from build123d import *

# Parameters (mm, degrees)
F0_W     = 62
F0_H     = 78
F0_W_2   = 8
F0_H_2   = 5
F1_DEPTH = 20
F2_W     = 54.3611720204
F2_H     = 31.5054729581
F3_DEPTH = 15


with BuildPart() as f1:
    # F0 (on Front) → F1 (new body, symmetric)
    with BuildSketch(Plane.XZ):
        Rectangle(F0_W, F0_H)
        with BuildLine():
            ThreePointArc((15.5, -16), (15.3535533906, -16.3535533906), (15, -16.5))
            Line((15, -16.5), (11.401754251, -16.5))
            ThreePointArc((11.401754251, -16.5), (9.7996656706, -18.0090196413), (8, -19.2759180474))
            Line((8, -19.2759180474), (8, -21))
            ThreePointArc((8, -21), (7.8535533906, -21.3535533906), (7.5, -21.5))
            Line((7.5, -21.5), (-7.5, -21.5))
            ThreePointArc((-7.5, -21.5), (-7.8535533906, -21.3535533906), (-8, -21))
            Line((-8, -21), (-8, -19.2759180474))
            ThreePointArc((-8, -19.2759180474), (-9.7996656706, -18.0090196413), (-11.401754251, -16.5))
            Line((-11.401754251, -16.5), (-15, -16.5))
            ThreePointArc((-15, -16.5), (-15.3535533906, -16.3535533906), (-15.5, -16))
            Line((-15.5, -16), (-15.5, -13.3574017484))
            Line((-15.5, -13.3574017484), (-17.7761566393, -11.5))
            Line((-17.7761566393, -11.5), (-19.75, -11.5))
            ThreePointArc((-19.75, -11.5), (-20.1035533906, -11.3535533906), (-20.25, -11))
            Line((-20.25, -11), (-20.25, -1))
            ThreePointArc((-20.25, -1), (-20.1035533906, -0.6464466094), (-19.75, -0.5))
            Line((-19.75, -0.5), (-17.7761566393, -0.5))
            Line((-17.7761566393, -0.5), (-15.5, 1.3574017484))
            Line((-15.5, 1.3574017484), (-15.5, 4))
            ThreePointArc((-15.5, 4), (-15.3535533906, 4.3535533906), (-15, 4.5))
            Line((-15, 4.5), (-11.6488967689, 4.5))
            Line((-11.6488967689, 4.5), (-9.7996656706, 6.0090196413))
            ThreePointArc((-9.7996656706, 6.0090196413), (-8.9223473587, 6.6744513732), (-8, 7.2759180474))
            Line((-8, 7.2759180474), (-8, 9.2156053036))
            ThreePointArc((-8, 9.2156053036), (-7.8535533906, 9.5691586942), (-7.5, 9.7156053036))
            Line((-7.5, 9.7156053036), (7.5, 9.7156053036))
            ThreePointArc((7.5, 9.7156053036), (7.8535533906, 9.5691586942), (8, 9.2156053036))
            Line((8, 9.2156053036), (8, 7.2759180474))
            ThreePointArc((8, 7.2759180474), (9.7996656706, 6.0090196413), (11.401754251, 4.5))
            Line((11.401754251, 4.5), (15, 4.5))
            ThreePointArc((15, 4.5), (15.3535533906, 4.3535533906), (15.5, 4))
            Line((15.5, 4), (15.5, 1.3574017484))
            Line((15.5, 1.3574017484), (17.7761566393, -0.5))
            Line((17.7761566393, -0.5), (19.75, -0.5))
            ThreePointArc((19.75, -0.5), (20.1035533906, -0.6464466094), (20.25, -1))
            Line((20.25, -1), (20.25, -11))
            ThreePointArc((20.25, -11), (20.1035533906, -11.3535533906), (19.75, -11.5))
            Line((19.75, -11.5), (17.7761566393, -11.5))
            Line((17.7761566393, -11.5), (15.5, -13.3574017484))
            Line((15.5, -13.3574017484), (15.5, -16))
        make_face(mode=Mode.SUBTRACT)
        with Locations((-19.3427710384, 30.9041780978)):
            Rectangle(F0_W_2, F0_H_2, mode=Mode.SUBTRACT)
        with Locations((19.3427710384, 30.9041780978)):
            Rectangle(F0_W_2, F0_H_2, mode=Mode.SUBTRACT)
    extrude(amount=F1_DEPTH, both=True)

    # F2 (on face) → F3 (join)
    with BuildSketch(Plane.XY.offset(39)):
        Rectangle(F2_W, F2_H)
    extrude(amount=-F3_DEPTH)


solid = f1.part
CAD build for the part. Positions are in the model's coordinates, mm. A direction names the side the tool comes from. Round coordinates to 2 decimals unless told otherwise and drop trailing zeros. Order: outer loops, then holes, each group sorted by start corner. A loop starts at its lowest first (then second) coordinate and runs counter-clockwise, first axis right, second up. Notation, with made-up numbers: (18, 83) -> (46, 83) arc R23 cw to (46, 121) -> close; hole circle Ø11 at (18, -15.75). An arc over 180 degrees is marked (long way). Write item = value, one per line. Start each with the question number.
(1) Cut at C-C, the plane x = 9.5. List the corners of the cut face in (y, z), then the cut area to 3 significant figures.
(2) Pin check, flat tips, straight feed: P1, Ø10, axis at x = -1, z = 0, coming from the -Y side; P2, Ø2.5, axis at x = 18, z = 31, coming from the +Y side. Stop position of each tip, or through.
(3) Cut at A-A, the plane x = -3.5. List the corners of the cut face in (y, z), then the cut area to 3 significant figures.
(4) Pull direction Z, two halves, no side cores. Call faces 4 (the flat face through (0, 0, -39)), 5 (the flat face through (19, 0, -11.5)): released by +Z, released by -Z, zero draft, split by the parting line, or undercut.
(5) Cut at D-D, the plane x = 16.5. List the corners of the cut face in (y, z).
(6) Probe line 1 (Z direction, x = -19, y = -17); line 2 (X direction, y = -13, z = -10); line 3 (Z direction, x = -13, y = 4). List the from-to ranges inside material, lowest first. Write a range as [from, to].
(7) Cut at B-B, the plane z = 30. List the corners of the cut face in (x, y).
(8) Which spindle directions (+Z, -Z, +X, -X, +Y, -Y) get a long thin tool onto all of the face, cutting with end or side? Do faces 1 (the flat face through (15.5, 0, -15)), 2 (the flat face through (-23.343, -18, 31)), 3 (the flat face through (19, 15.753, 31)). Say none if no direction does.
Model answer:
q1.outline = (-20, -39) -> (20, -39) -> (20, -18.25) -> (-20, -18.25) -> close; (-20, 6.25) -> (20, 6.25) -> (20, 39) -> (-20, 39) -> close
q1.area = 2,140 mm2
q2.P1 = through
q2.P2 = 15.75
q3.outline = (-20, -39) -> (20, -39) -> (20, -21.5) -> (-20, -21.5) -> close; (-20, 9.72) -> (20, 9.72) -> (20, 39) -> (-20, 39) -> close
q3.area = 1,870 mm2
q4.face_4 = released by -Z
q4.face_5 = undercut
q5.outline = (-20, -39) -> (20, -39) -> (20, -12.54) -> (-20, -12.54) -> close; (-20, 0.54) -> (20, 0.54) -> (20, 28.4) -> (15.75, 28.4) -> (15.75, 33.4) -> (20, 33.4) -> (20, 39) -> (-20, 39) -> (-20, 33.4) -> (-15.75, 33.4) -> (-15.75, 28.4) -> (-20, 28.4) -> close
q6.line_1 = [-39, -11.5], [-0.5, 28.4], [33.4, 39]
q6.line_2 = [-31, -20.25], [20.25, 31]
q6.line_3 = [-39, -16.5], [4.5, 39]
q7.outline = (-31, -20) -> (-23.34, -20) -> (-23.34, -15.75) -> (-15.34, -15.75) -> (-15.34, -20) -> (15.34, -20) -> (15.34, -15.75) -> (23.34, -15.75) -> (23.34, -20) -> (31, -20) -> (31, 20) -> (23.34, 20) -> (23.34, 15.75) -> (15.34, 15.75) -> (15.34, 20) -> (-15.34, 20) -> (-15.34, 15.75) -> (-23.34, 15.75) -> (-23.34, 20) -> (-31, 20) -> close
q8.face_1 = +Y, -Y
q8.face_2 = -Y
q8.face_3 = +Y
